The listing builds one solid part. Answer for the finished solid, in the listing's coordinates (mm). Round coordinates to 2 decimals unless told otherwise and drop trailing zeros. Write each loop counter-clockwise with the first axis right and the second up, starting at its lowest first coordinate (ties: lowest second). Pieces come first, ordered by that corner, then holes. Notation, with made-up numbers: M 2,77 L 15,77 A24 ccw 15,99 Z; hole C 85.25,70.5 d4. An arc over 180 degrees is marked long. One line per item, written item: value. Start each with the question number.
(1) Section C-C (z = 5.25) is taken. State how many separate pieces and enclosed holes the cut face has, plus the area to 3 significant figures.
(2) Section B-B (y = 79.5) is taken. Determine the outline of the cut face in (x, z).
(3) Consider probe 1 along Y at (x, z) = (71, 2.5); probe 2 along X at (y, z) = (69.85, 3.75); probe 3 along X at (y, z) = (12.7, 1.5). Determine where each line is inside the solid, lowest interval first.
(4) Section A-A (x = 81.5) is taken. Determine the outline of the cut face in (y, z), plus the area to 3 significant figures.
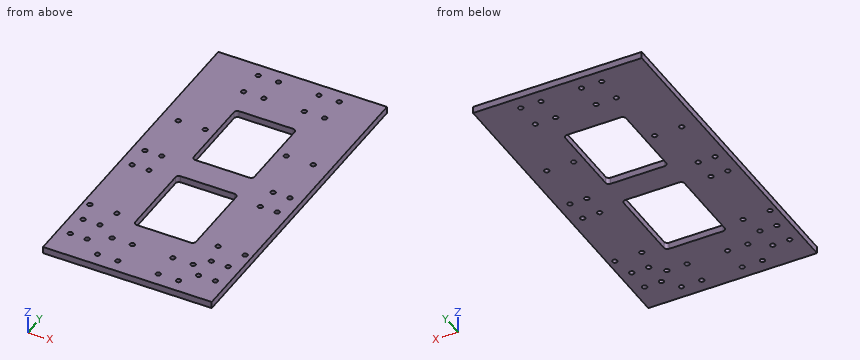
Autodesk Inventor part; units mm, degrees
ref_plane "YZ Plane" through (0, 0, 0) normal (1, 0, 0) x (0, 1, 0)
ref_plane "XZ Plane" through (0, 0, 0) normal (0, 1, 0) x (-1, 0, 0)
ref_plane "XY Plane" through (0, 0, 0) normal (0, 0, 1) x (1, 0, 0)
sketch "Sketch1" plane through (0, 0, 0) normal (0, 0, 1) x (1, 0, 0)
  line L0 (0, 0) -> (158.75, 0)
  line L1 (158.75, 0) -> (158.75, 304.8)
  line L2 (158.75, 304.8) -> (0, 304.8)
  line L3 (0, 304.8) -> (0, 0)
  dimension "d0" = 158.75
  dimension "d1" = 304.8
extrude "Extrusion1" add sketch "Sketch1" along normal blind 6.35
sketch "Sketch2" plane through (0, 0, 0) normal (0, 0, -1) x (-1, 0, 0)
  circle A0 centre (-117.475, 205.8824) radius 2.4638
  line L0 (-177.2766, 228.1074) -> (-172.9586, 228.1074)
  circle A1 centre (-142.875, 205.8824) radius 2.4638
  circle A2 centre (-41.275, 205.8824) radius 2.4638
  circle A3 centre (-15.875, 205.8824) radius 2.4638
  circle A4 centre (-147.6375, 26.9875) radius 2.4638
  circle A5 centre (-131.7625, 26.9875) radius 2.4638
  circle A6 centre (-131.7625, 49.2125) radius 2.4638
  circle A7 centre (-147.6375, 49.2125) radius 2.4638
  circle A8 centre (-26.9875, 26.9875) radius 2.4638
  circle A9 centre (-11.1125, 26.9875) radius 2.4638
  circle A10 centre (-11.1125, 49.2125) radius 2.4638
  circle A11 centre (-26.9875, 49.2125) radius 2.4638
  circle A12 centre (-11.1125, 156.6699) radius 2.4638
  circle A13 centre (-11.1125, 134.4449) radius 2.4638
  circle A14 centre (-26.9875, 134.4449) radius 2.4638
  circle A15 centre (-26.9875, 156.6699) radius 2.4638
  circle A16 centre (-147.6375, 134.4449) radius 2.4638
  circle A17 centre (-131.7625, 134.4449) radius 2.4638
  circle A18 centre (-147.6375, 156.6699) radius 2.4638
  circle A19 centre (-131.7625, 156.6699) radius 2.4638
  point P0 (0, 0)
sketch "Sketch3" plane through (0, 0, 0) normal (0, 0, -1) x (-1, 0, 0)
  line L0 (47.625, 49.2116) -> (-206.375, 49.2116)
  point P0 (0, 0)
  point P1 (-142.875, 205.8824)
  point P2 (-117.475, 205.8824)
  point P3 (-131.7625, 156.6699)
  point P4 (-147.6375, 156.6699)
  point P5 (-147.6375, 134.4449)
  point P6 (-131.7625, 134.4449)
  point P7 (-147.6375, 49.2125)
  point P8 (-131.7625, 49.2125)
  point P9 (-131.7625, 26.9875)
  point P10 (-147.6375, 26.9875)
  point P11 (-26.9875, 26.9875)
  point P12 (-11.1125, 26.9875)
  point P13 (-11.1125, 49.2125)
  point P14 (-26.9875, 49.2125)
  point P15 (-26.9875, 134.4449)
  point P16 (-11.1125, 134.4449)
  point P17 (-11.1125, 156.6699)
  point P18 (-26.9875, 156.6699)
  point P19 (-41.275, 205.8824)
  point P20 (-15.875, 205.8824)
hole "Hole1" at (142.875, 205.8824, 0) at (117.475, 205.8824, 0) at (41.275, 205.8824, 0) at (15.875, 205.8824, 0) at (26.9875, 156.6699, 0) at (11.1125, 156.6699, 0) at (11.1125, 134.4449, 0) at (26.9875, 134.4449, 0) at (131.7625, 156.6699, 0) at (147.6375, 156.6699, 0) at (131.7625, 134.4449, 0) at (147.6375, 134.4449, 0) at (147.6375, 49.2125, 0) at (131.7625, 49.2125, 0) at (131.7625, 26.9875, 0) at (147.6375, 26.9875, 0) at (26.9875, 26.9875, 0) at (11.1125, 26.9875, 0) at (11.1125, 49.2125, 0) at (26.9875, 49.2125, 0) direction (0, 0, 1) diameter 4.4958 depth 25.4 tip angle 118
sketch "Sketch4" plane through (0, 0, 0) normal (0, 0, -1) x (-1, 0, 0)
  circle A0 centre (-11.1125, 49.2125) radius 2.2479
  circle A1 centre (-26.9875, 26.9875) radius 2.2479
  circle A2 centre (-131.7625, 26.9875) radius 2.2479
  circle A3 centre (-147.6375, 49.2125) radius 2.2479
  circle A4 centre (-131.7625, 134.4449) radius 2.2479
  circle A5 centre (-131.7625, 156.6699) radius 2.2479
  circle A6 centre (-11.1125, 134.4449) radius 2.2479
  circle A7 centre (-26.9875, 156.6699) radius 2.2479
  circle A8 centre (-41.275, 205.8824) radius 2.2479
  circle A9 centre (-142.875, 205.8824) radius 2.2479
  circle A10 centre (-117.475, 205.8824) radius 2.2479
  circle A11 centre (-15.875, 205.8824) radius 2.2479
  circle A12 centre (-11.1125, 156.6699) radius 2.2479
  circle A13 centre (-26.9875, 134.4449) radius 2.2479
  circle A14 centre (-147.6375, 156.6699) radius 2.2479
  circle A15 centre (-147.6375, 134.4449) radius 2.2479
  circle A16 centre (-131.7625, 49.2125) radius 2.2479
  circle A17 centre (-147.6375, 26.9875) radius 2.2479
  circle A18 centre (-11.1125, 26.9875) radius 2.2479
  circle A19 centre (-26.9875, 49.2125) radius 2.2479
  line L0 (0, 0) -> (-158.75, 0)
  line L1 (0, 304.8) -> (0, 0)
  line L2 (-158.75, 304.8) -> (0, 304.8)
  line L3 (-158.75, 0) -> (-158.75, 304.8)
  line L4 (-82.55, 718.8359) -> (-82.55, -134.6309)
  line L5 (0, 0) -> (-158.75, 0)
  point P0 (-120.65, 38.1)
  point P1 (-120.65, 12.7)
  point P2 (-44.45, 38.1)
  point P3 (-44.45, 12.7)
  point P4 (-101.6, 38.1)
  point P5 (-63.5, 38.1)
  point P6 (-63.5, 12.7)
  point P7 (-101.6, 12.7)
  dimension "d11" = 19.05
  dimension "d12" = 19.05
  dimension "d13" = 19.05
  dimension "d14" = 19.05
  dimension "d15" = 19.05
  dimension "d16" = 19.05
  dimension "d17" = 19.05
  dimension "d18" = 19.05
  dimension "d19" = 25.4
  dimension "d20" = 25.4
  dimension "d21" = 12.7
  dimension "d22" = 12.7
  dimension "d23" = 12.7
  dimension "d24" = 12.7
hole "Hole2" at (120.65, 38.1, 0) at (120.65, 12.7, 0) at (44.45, 38.1, 0) at (44.45, 12.7, 0) at (101.6, 38.1, 0) at (63.5, 38.1, 0) at (63.5, 12.7, 0) at (101.6, 12.7, 0) direction (0, 0, 1) diameter 4.4958 depth 25.4 tip angle 118
ref_plane "Work Plane1" through (0, 152.4, 0) normal (0, 1, 0) x (1, 0, 0)
mirror "Mirror1" about plane through (0, 152.4, 0) normal (0, 1, 0) of "Hole2"
sketch "Sketch5" plane through (0, 0, 0) normal (0, 0, -1) x (-1, 0, 0)
  line L0 (-107.95, 241.3) -> (-50.8, 241.3)
  line L1 (-50.8, 241.3) -> (-50.8, 63.5)
  line L2 (-50.8, 63.5) -> (-107.95, 63.5)
  line L3 (-107.95, 63.5) -> (-107.95, 241.3)
  line L4 (0, 0) -> (-158.75, 0)
  line L5 (-158.75, 304.8) -> (0, 304.8)
  line L6 (0, 304.8) -> (0, 0)
  line L7 (-158.75, 0) -> (-158.75, 304.8)
  dimension "d32" = 63.5
  dimension "d33" = 63.5
  dimension "d34" = 50.8
  dimension "d35" = 50.8
extrude "Extrusion2" cut sketch "Sketch5" against normal blind 6.35 contours L0 L1 L2 L3
sketch "Sketch6" plane through (0, 0, 0) normal (0, 0, -1) x (-1, 0, 0)
  line L0 (-107.95, 63.5) -> (-107.95, 241.3)
  line L1 (-50.8, 241.3) -> (-50.8, 63.5)
  line L2 (-107.95, 165.1) -> (-50.8, 165.1)
  line L3 (-50.8, 165.1) -> (-50.8, 139.7)
  line L4 (-50.8, 139.7) -> (-107.95, 139.7)
  line L5 (-107.95, 139.7) -> (-107.95, 165.1)
  line L6 (-212.7319, 152.4) -> (35.4553, 152.4)
  point P0 (0, 0)
  dimension "d38" = 12.7
  dimension "d39" = 12.7
extrude "Extrusion3" add sketch "Sketch6" against normal up to surface (6.35 mm away)
fillet "Fillet1" radius 3.175 4 edges at (50.8, 241.3, 3.175) (107.95, 241.3, 3.175) (107.95, 165.1, 3.175) (50.8, 165.1, 3.175)
fillet "Fillet2" radius 3.175 4 edges at (107.95, 139.7, 3.175) (50.8, 139.7, 3.175) (107.95, 63.5, 3.175) (50.8, 63.5, 3.175)
sketch "Sketch7" plane through (0, 0, 0) normal (0, 0, -1) x (-1, 0, 0)
  line L0 (0, 0) -> (-158.75, 0)
  line L1 (0, 304.8) -> (0, 0)
  line L2 (-158.75, 0) -> (-158.75, 304.8)
  point P0 (-127, 69.85)
  point P1 (-152.4, 69.85)
  point P2 (-6.35, 69.85)
  point P3 (-31.75, 69.85)
  dimension "d44" = 25.4
  dimension "d45" = 69.85
  dimension "d46" = 69.85
  dimension "d47" = 69.85
  dimension "d48" = 69.85
  dimension "d49" = 25.4
  dimension "d50" = 6.35
  dimension "d51" = 6.35
hole "Hole3" at (127, 69.85, 0) at (152.4, 69.85, 0) at (6.35, 69.85, 0) at (31.75, 69.85, 0) direction (0, 0, 1) diameter 4.4958 depth 25.4 tip angle 118
equation "\"d39\" = d38"
properties part number "Gripper Back"
Recorded:
1. separate pieces: 1
1. enclosed holes: 42
1. area: 39,100 mm2
2. outline: M 0,0 L 50.8,0 L 50.8,6.35 L 0,6.35 Z; M 107.95,0 L 158.75,0 L 158.75,6.35 L 107.95,6.35 Z
3. probe 1: y = 0 to 63.5, 139.7 to 165.1, 241.3 to 304.8
3. probe 2: x = 0 to 4.1, 8.6 to 29.5, 34 to 50.8, 107.95 to 124.75, 129.25 to 150.15, 154.65 to 158.75
3. probe 3: x = 0 to 42.2, 46.7 to 61.25, 65.75 to 99.35, 103.85 to 118.4, 122.9 to 158.75
4. outline: M 0,0 L 63.5,0 L 63.5,6.35 L 0,6.35 Z; M 139.7,0 L 165.1,0 L 165.1,6.35 L 139.7,6.35 Z; M 241.3,0 L 304.8,0 L 304.8,6.35 L 241.3,6.35 Z
4. area: 968 mm2
